Answer from the drawing. Dimensions are ordinates in mm from the lowest x, y and z of the part. Round coordinates to 2 decimals unless told otherwise and drop trailing zeros. Write each loop counter-clockwise with the first axis right and the second up, starting at its lowest first coordinate (ties: lowest second). Pieces come first, ordered by that corner, then holes. Notation, with made-up numbers: (-39, -8.75) - (-8, -8.75) arc R16 cw to (-8, 6.25) - close; hole circle Ø5 at (12.25, -10). An arc over 180 degrees is marked (long way). One line per item, written item: value. Start each with the question number.
(1) Find the intervals of material crossed by L1, parallel to Y at x = 50, z = 27; L2, parallel to Y at x = 36.5, z = 26.5; L3, parallel to X at y = 54, z = 17, in increasing order.
(2) Flat-ended cylindrical pins translate along their axes: pin 1 Ø2 at (x, z) = (17.5, 45) entering from +Y; pin 2 Ø6 at (x, z) = (26, 37.5) entering from -Y; pin 3 Ø5 at (x, z) = (41, 40.5) entering from -Y; pin 4 Ø8 at (y, z) = (54, 28.5) entering from -X. Find the tip coordinate at first contact, or state that the pin passes through.
(3) The mould has two halves that part along Y. Classify the marked faces 1, 2 and 3: +Y half, -Y half, draft (parallel to the pull), parting line (faces both ways), or undercut.
(4) A cutting plane is placed at C-C, the plane z = 23. Determine the outline of the cut face in (x, y).
(5) A cutting plane is placed at A-A, the plane x = 50.8. Determine the outline of the cut face in (y, z).
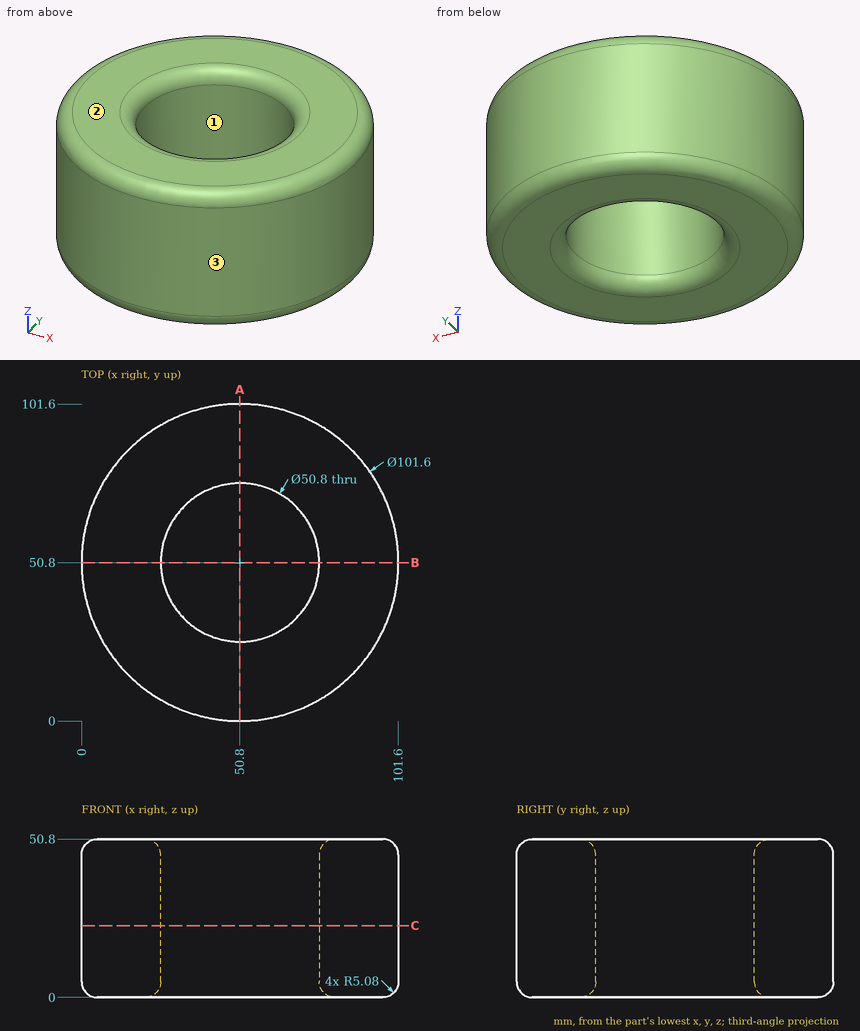
Here are the results:
1. L1: 0.01 to 25.41, 76.19 to 101.59
1. L2: 2.05 to 29.81, 71.79 to 99.55
1. L3: 0.1 to 25.6, 76 to 101.5
2. pin 1: y = 90.01
2. pin 2: y = 4.92
2. pin 3: y = 0.53
2. pin 4: x = 0
3. face 1: undercut
3. face 2: draft
3. face 3: parting line
4. outline: circle Ø101.6 at (50.8, 50.8); hole circle Ø50.8 at (50.8, 50.8)
5. outline: (0, 5.08) arc R5.08 ccw to (5.08, 0) - (20.32, 0) arc R5.08 ccw to (25.4, 5.08) - (25.4, 45.72) arc R5.08 ccw to (20.32, 50.8) - (5.08, 50.8) arc R5.08 ccw to (0, 45.72) - close; (76.2, 5.08) arc R5.08 ccw to (81.28, 0) - (96.52, 0) arc R5.08 ccw to (101.6, 5.08) - (101.6, 45.72) arc R5.08 ccw to (96.52, 50.8) - (81.28, 50.8) arc R5.08 ccw to (76.2, 45.72) - close
